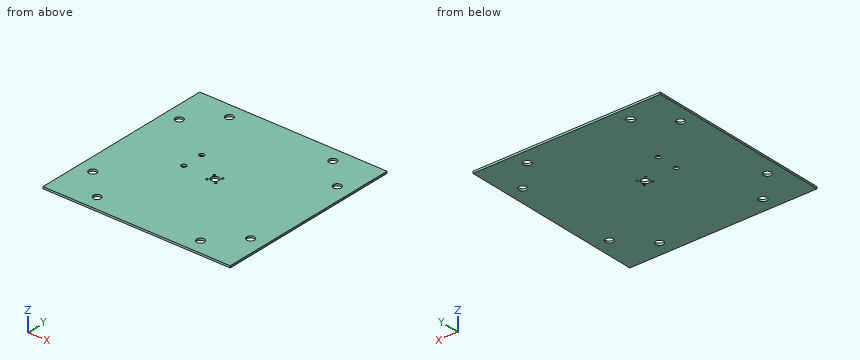
from build123d import *

# Parameters (mm, degrees)
F0_W     = 304.8
F0_H     = 304.8
F0_R     = 6.35
F0_R_2   = 1.7526
F0_R_3   = 3.96875
F1_DEPTH = 3.175


with BuildPart() as f1:
    # F0 (on Top) → F1 (new body)
    with BuildSketch(Plane.XY):
        Rectangle(F0_W, F0_H)
        with Locations((-84.1375, -128.5875)):
            Circle(F0_R, mode=Mode.SUBTRACT)
        with Locations((-128.5875, -84.1375)):
            Circle(F0_R, mode=Mode.SUBTRACT)
        with Locations((-6.914797, -6.914797)):
            Circle(F0_R_2, mode=Mode.SUBTRACT)
        with Locations((84.13242, -128.5875)):
            Circle(F0_R, mode=Mode.SUBTRACT)
        with Locations((128.5875, -84.1375)):
            Circle(F0_R, mode=Mode.SUBTRACT)
        with Locations((6.914797, -6.914797)):
            Circle(F0_R_2, mode=Mode.SUBTRACT)
        with Locations((-50.8, 0)):
            Circle(F0_R_3, mode=Mode.SUBTRACT)
        with Locations((-50.8, 34.925)):
            Circle(F0_R_3, mode=Mode.SUBTRACT)
        with Locations((-6.914797, 6.914797)):
            Circle(F0_R_2, mode=Mode.SUBTRACT)
        with Locations((-128.5875, 84.1375)):
            Circle(F0_R, mode=Mode.SUBTRACT)
        with Locations((-84.1375, 128.5875)):
            Circle(F0_R, mode=Mode.SUBTRACT)
        Circle(F0_R, mode=Mode.SUBTRACT)
        with Locations((6.914797, 6.914797)):
            Circle(F0_R_2, mode=Mode.SUBTRACT)
        with Locations((128.5875, 84.1375)):
            Circle(F0_R, mode=Mode.SUBTRACT)
        with Locations((84.1375, 128.6002)):
            Circle(F0_R, mode=Mode.SUBTRACT)
    extrude(amount=F1_DEPTH)


solid = f1.part
Design review of the part built by this model. Coordinates are the model's own, in mm. Give positions to 0.01 mm unless a question says otherwise; leave off trailing zeros. Write each loop counter-clockwise with the first axis right and the second up, starting at its lowest first coordinate (ties: lowest second). Pieces come first, ordered by that corner, then holes. Notation, with made-up numbers: M 53.25,-4 L 99.25,-4 A18 ccw 99.25,16 Z; hole C 68,56 d1. An arc over 180 degrees is marked long. Answer as a JSON object with one key per item and string values. Group by question number.
1) For line 1 along X through (y, z) = (-84, 0.55); line 2 along Y through (x, z) = (-50.8, 0.7); line 3 along X through (y, z) = (80, 2.55), list the stretches that pass through material, from the lowest coordinate up.
2) We need section B-B (y = 0). Give the boundary of the cut face in (x, z) (3 decimals), and give its area (3 significant figures).
3) Clearance check with a flat-ended pin moving along its axis: pin 1 Ø2 at (x, y) = (-6.91, 6.91) entering from +Z. State where the tip first meets the part, or that it passes through.
4) We need section A-A (x = -50.8). Give the boundary of the cut face in (y, z) (3 decimals), and give its area (3 significant figures).
5) We need section C-C (x = 0). Give the boundary of the cut face in (y, z) (3 decimals), and give its area (3 significant figures).
Answer key:
{
 "1": {"line 1": "x = -152.4 to -134.94, -122.24 to 122.24, 134.94 to 152.4", "line 2": "y = -152.4 to -3.97, 3.97 to 30.96, 38.89 to 152.4", "line 3": "x = -152.4 to -133.4, -123.77 to 123.77, 133.4 to 152.4"},
 "2": {"outline": "M -152.4,0 L -54.769,0 L -54.769,3.175 L -152.4,3.175 Z; M -46.831,0 L -6.35,0 L -6.35,3.175 L -46.831,3.175 Z; M 6.35,0 L 152.4,0 L 152.4,3.175 L 6.35,3.175 Z", "area": "902 mm²"},
 "3": {"pin 1": "passes through"},
 "4": {"outline": "M -152.4,0 L -3.969,0 L -3.969,3.175 L -152.4,3.175 Z; M 3.969,0 L 30.956,0 L 30.956,3.175 L 3.969,3.175 Z; M 38.894,0 L 152.4,0 L 152.4,3.175 L 38.894,3.175 Z", "area": "917 mm²"},
 "5": {"outline": "M -152.4,0 L -6.35,0 L -6.35,3.175 L -152.4,3.175 Z; M 6.35,0 L 152.4,0 L 152.4,3.175 L 6.35,3.175 Z", "area": "927 mm²"}
}
